from build123d import *

# Parameters (mm, degrees)
BOSS_EXTRUDE1_DEPTH = 1.5875
SKETCH2_R           = 1.5875
CUT_EXTRUDE1_DEPTH  = 2.54
LPATTERN2_COUNT     = 2
LPATTERN2_PITCH     = 38.1
SKETCH3_W           = 6.35
SKETCH3_H           = 34.925
CUT_EXTRUDE2_DEPTH  = 2.54


with BuildPart() as part:
    # Sketch1 → Boss-Extrude1 (new body)
    with BuildSketch(Plane.XY):
        Polygon((0, 0), (0, 34.925), (34.925, 34.925), (63.5, 6.35), (63.5, 0), align=None)
    extrude(amount=BOSS_EXTRUDE1_DEPTH)

    # Sketch2 → Cut-Extrude1 (cut)
    with BuildSketch(Plane.XY.offset(1.5875)):
        with Locations((12.7, 3.175)):
            Circle(SKETCH2_R)
    cut_extrude1 = extrude(amount=-CUT_EXTRUDE1_DEPTH, mode=Mode.SUBTRACT)

    # LPattern2: Cut-Extrude1 ×2
    with Locations(*[(i * LPATTERN2_PITCH, 0, 0) for i in range(1, LPATTERN2_COUNT)]):
        add(cut_extrude1, mode=Mode.SUBTRACT)

    # Sketch3 → Cut-Extrude2 (cut)
    with BuildSketch(Plane.XY.offset(1.5875)):
        with Locations((3.175, 17.4625)):
            Rectangle(SKETCH3_W, SKETCH3_H)
    extrude(amount=-CUT_EXTRUDE2_DEPTH, mode=Mode.SUBTRACT)


solid = part.part
For this review, take the finished solid that the model builds, in its own axes (mm). Round coordinates to 2 decimals unless told otherwise and drop trailing zeros. Order: outer loops, then holes, each group sorted by start corner. A loop starts at its lowest first (then second) coordinate and runs counter-clockwise, first axis right, second up. Notation, with made-up numbers: M 29.25,-35.5 L 74.25,-35.5 A16 ccw 74.25,-17.5 Z; hole C -28.75,28 d3. An arc over 180 degrees is marked long. Use a Markdown table: item, result. Add a question column.
Item 1: Mouldability with a two-part tool opening along Y and no side actions: class faces 1 (the cylindrical face through (14.2, 3.7, 0.8)), 2 (the flat face through (35, 0, 1)), 3 (the flat face through (20, 34.925, 1)), 4 (the flat face through (6.35, 17, 1)) as released by +Y, released by -Y, zero draft, split by the parting line, or undercut.
Item 2: Add section A-A, the plane x = 12.7. Give the boundary of the cut face in (y, z) (1 decimal), then the cut area to 3 significant figures.
Item 3: Insertion check: pin 1 (5 mm diameter, centred on x = 12.7, y = 3.175, fed in from +Z). The pin has a flat end and moves straight along its axis. Give the tip position at first contact, or say it passes through.
Item 4: Add section D-D, the plane y = 21. Give the boundary of the cut face in (x, z), then the cut area to 3 significant figures.
Item 5: Add section C-C, the plane z = 0.55. State how many separate pieces and enclosed holes the cut face has, then the cut area to 3 significant figures.
Item 6: To check wall thickness, follow line 1 along Y through (x, z) = (12.7, 0.4) (1 decimal); line 2 along Y through (x, z) = (50.8, 1.3); line 3 along X through (y, z) = (20, 0.7). State the ranges of each line that lie inside material, in increasing order.
Item 7: Add section B-B, the plane x = 50.8. Give the boundary of the cut face in (y, z), then the cut area to 3 significant figures.
Geometry results:
| question | item | result |
|---|---|---|
| 1 | face 1 | undercut |
| 1 | face 2 | released by -Y |
| 1 | face 3 | released by +Y |
| 1 | face 4 | zero draft |
| 2 | outline | M 0,0 L 1.6,0 L 1.6,1.6 L 0,1.6 Z; M 4.8,0 L 34.9,0 L 34.9,1.6 L 4.8,1.6 Z |
| 2 | area | 50.4 mm² |
| 3 | pin 1 | stops at z = 1.59 |
| 4 | outline | M 6.35,0 L 48.85,0 L 48.85,1.59 L 6.35,1.59 Z |
| 4 | area | 67.5 mm² |
| 5 | separate pieces | 1 |
| 5 | enclosed holes | 2 |
| 5 | area | 1,570 mm² |
| 6 | line 1 | y = 0 to 1.6, 4.8 to 34.9 |
| 6 | line 2 | y = 0 to 1.59, 4.76 to 19.05 |
| 6 | line 3 | x = 6.35 to 49.85 |
| 7 | outline | M 0,0 L 1.59,0 L 1.59,1.59 L 0,1.59 Z; M 4.76,0 L 19.05,0 L 19.05,1.59 L 4.76,1.59 Z |
| 7 | area | 25.2 mm² |
